Autodesk Inventor part; units mm, degrees
ref_plane "YZ Plane" through (0, 0, 0) normal (1, 0, 0) x (0, 1, 0)
ref_plane "XZ Plane" through (0, 0, 0) normal (0, 1, 0) x (-1, 0, 0)
ref_plane "XY Plane" through (0, 0, 0) normal (0, 0, 1) x (1, 0, 0)
sketch "Sketch1" plane through (0, 0, 0) normal (0, 0, 1) x (1, 0, 0)
  line L0 (0, 0) -> (254, 0)
  line L1 (254, 0) -> (254, 279.4)
  line L2 (254, 279.4) -> (0, 279.4)
  line L3 (0, 279.4) -> (0, 0)
  line L4 (92.075, 228.6) -> (117.475, 228.6)
  line L5 (117.475, 228.6) -> (117.475, 50.8)
  line L6 (117.475, 50.8) -> (92.075, 50.8)
  line L7 (92.075, 50.8) -> (92.075, 228.6)
  line L8 (136.525, 228.6) -> (161.925, 228.6)
  line L9 (161.925, 228.6) -> (161.925, 50.8)
  line L10 (161.925, 50.8) -> (136.525, 50.8)
  line L11 (136.525, 50.8) -> (136.525, 228.6)
  line L12 (117.475, 228.6) -> (136.525, 228.6)
  point P0 (127, 228.6)
  point P1 (127, 279.4)
  dimension "d0" = 254
  dimension "d1" = 279.4
  dimension "d2" = 19.05
  dimension "d3" = 25.4
  dimension "d4" = 25.4
  dimension "d5" = 50.8
  dimension "d6" = 50.8
extrude "Extrusion1" add sketch "Sketch1" along normal blind 2.286
fillet "Fillet1" radius 1.5875 8 edges at (92.075, 50.8, 1.143) (117.475, 50.8, 1.143) (136.525, 50.8, 1.143) (161.925, 50.8, 1.143) (161.925, 228.6, 1.143) (136.525, 228.6, 1.143) (117.475, 228.6, 1.143) (92.075, 228.6, 1.143)
sketch "Sketch2" plane through (0, 0, 2.286) normal (0, 0, 1) x (1, 0, 0)
  line L0 (9.525, 269.875) -> (34.925, 269.875)
  line L1 (34.925, 269.875) -> (34.925, 231.775)
  line L2 (34.925, 231.775) -> (9.525, 231.775)
  line L3 (9.525, 231.775) -> (9.525, 269.875)
  line L4 (219.075, 269.875) -> (244.475, 269.875)
  line L5 (244.475, 269.875) -> (244.475, 231.775)
  line L6 (244.475, 231.775) -> (219.075, 231.775)
  line L7 (219.075, 231.775) -> (219.075, 269.875)
  line L8 (0, 279.4) -> (0, 0)
  line L9 (254, 0) -> (254, 279.4)
  line L10 (254, 279.4) -> (0, 279.4)
  dimension "d10" = 9.525
  dimension "d11" = 9.525
  dimension "d12" = 9.525
  dimension "d13" = 25.4
  dimension "d14" = 38.1
extrude "Extrusion2" cut sketch "Sketch2" against normal through all
equation "\"d4\" = d3"
equation "\"d11\" = d10"
properties part number "Interior Frame"
Can you work these out from the model? Positions are in its coordinate system, mm. Give positions to 0.01 mm unless a question says otherwise; leave off trailing zeros. Write each loop counter-clockwise with the first axis right and the second up, starting at its lowest first coordinate (ties: lowest second). Pieces come first, ordered by that corner, then holes. Notation, with made-up numbers: (14.5, -7.5) - (73.5, -7.5) arc R8 cw to (73.5, -1.5) - close; hole circle Ø2 at (44.25, 20). An arc over 180 degrees is marked (long way). Write item = value, one per line. Start each with the question number.
1. Imagine slicing it at B-B (y = 130.5). Please give me the cut outline in (x, z) (3 decimals).
2. Imagine slicing it at C-C (z = 1.25). Please give me the cut outline in (x, y) (1 decimal), and give its area (3 significant figures).
3. Imagine slicing it at A-A (x = 229.5). Please give me the cut outline in (y, z) (3 decimals), and give its area (3 significant figures).
4. Please list where these lines run through material, in increasing order: line 1 (X direction, y = 268, z = 1.1) (3 decimals); line 2 (X direction, y = 139, z = 0.3) (3 decimals); line 3 (Y direction, x = 112.5, z = 1.35).
Worked answers:
q1.outline = (0, 0) - (92.075, 0) - (92.075, 2.286) - (0, 2.286) - close; (117.475, 0) - (136.525, 0) - (136.525, 2.286) - (117.475, 2.286) - close; (161.925, 0) - (254, 0) - (254, 2.286) - (161.925, 2.286) - close
q2.outline = (0, 0) - (254, 0) - (254, 279.4) - (0, 279.4) - close; hole (9.5, 231.8) - (34.9, 231.8) - (34.9, 269.9) - (9.5, 269.9) - close; hole (92.1, 52.4) arc R1.6 ccw to (93.7, 50.8) - (115.9, 50.8) arc R1.6 ccw to (117.5, 52.4) - (117.5, 227) arc R1.6 ccw to (115.9, 228.6) - (93.7, 228.6) arc R1.6 ccw to (92.1, 227) - close; hole (136.5, 52.4) arc R1.6 ccw to (138.1, 50.8) - (160.3, 50.8) arc R1.6 ccw to (161.9, 52.4) - (161.9, 227) arc R1.6 ccw to (160.3, 228.6) - (138.1, 228.6) arc R1.6 ccw to (136.5, 227) - close; hole (219.1, 231.8) - (244.5, 231.8) - (244.5, 269.9) - (219.1, 269.9) - close
q2.area = 60,000 mm2
q3.outline = (0, 0) - (231.775, 0) - (231.775, 2.286) - (0, 2.286) - close; (269.875, 0) - (279.4, 0) - (279.4, 2.286) - (269.875, 2.286) - close
q3.area = 552 mm2
q4.line_1 = 0 to 9.525, 34.925 to 219.075, 244.475 to 254
q4.line_2 = 0 to 92.075, 117.475 to 136.525, 161.925 to 254
q4.line_3 = 0 to 50.8, 228.6 to 279.4
